```python
from build123d import *

# Parameters (mm, degrees)
BASE_FLANGE1_DEPTH = 2
HEM1_START         = -30
HEM1_DEPTH         = 10
HEM1_START_2       = 20
HEM1_2_DEPTH       = 10
SKETCH14_R         = 2
CUT_EXTRUDE1_DEPTH = 10
CHAMFER1_SIZE      = 1


# Read off the part's stored shape, not the designer's step: Hem1
# Sheet-metal steps are written as plain solids
with BuildPart() as part:
    # Sketch1 → Base-Flange1 (new body)
    with BuildSketch(Plane(origin=(0, 0, 0), x_dir=(1, 0, 0), z_dir=(0, 1, 0))):
        with BuildLine():
            Line((20, -15), (30, -15))
            Line((30, -15), (30, 12))
            ThreePointArc((30, 12), (29.121320344, 14.121320344), (27, 15))
            Line((27, 15), (-27, 15))
            ThreePointArc((-27, 15), (-29.121320344, 14.121320344), (-30, 12))
            Line((-30, 12), (-30, -15))
            Line((-30, -15), (-20, -15))
            Line((-20, -15), (-20, 2))
            ThreePointArc((-20, 2), (-19.121320344, 4.121320344), (-17, 5))
            Line((-17, 5), (17, 5))
            ThreePointArc((17, 5), (19.121320344, 4.121320344), (20, 2))
            Line((20, 2), (20, -15))
        make_face()
    extrude(amount=-BASE_FLANGE1_DEPTH)

    # Hem1 outline → Hem1 (add)
    with BuildSketch(Plane.YZ.offset(HEM1_START)):
        with BuildLine():
            Line((2.038247626, 12.343703978), (1.520609536, 10.411852325))
            ThreePointArc((1.520609536, 10.411852325), (6.518428366, 17.891616788), (-2, 15))
            Line((-2, 15), (0, 15))
            ThreePointArc((0, 15), (4.931721686, 16.67409393), (2.038247626, 12.343703978))
        make_face()
    extrude(amount=HEM1_DEPTH)

    # Hem1 2 outline → Hem1 2 (add)
    with BuildSketch(Plane.YZ.offset(HEM1_START_2)):
        with BuildLine():
            Line((2.038247626, 12.343703978), (1.520609536, 10.411852325))
            ThreePointArc((1.520609536, 10.411852325), (6.518428366, 17.891616788), (-2, 15))
            Line((-2, 15), (0, 15))
            ThreePointArc((0, 15), (4.931721686, 16.67409393), (2.038247626, 12.343703978))
        make_face()
    extrude(amount=HEM1_2_DEPTH)

    # Sketch14 → Cut-Extrude1 (cut)
    with BuildSketch(Plane(origin=(0, 0, 0), x_dir=(1, 0, 0), z_dir=(0, 1, 0))):
        with Locations(Location((0, 10, 0), (0, 0, 270))):
            Circle(SKETCH14_R)
        with Locations(Location((-25, -5, 0), (0, 0, 270))):
            Circle(SKETCH14_R)
        with Locations(Location((25, -5, 0), (0, 0, 270))):
            Circle(SKETCH14_R)
    extrude(amount=-CUT_EXTRUDE1_DEPTH, mode=Mode.SUBTRACT)

    # Chamfer1
    chamfer1_edges = [part.edges().sort_by_distance(p)[0] for p in [
        (0, 0, -12),
        (-25, 0, 3),
        (25, 0, 3),
    ]]
    chamfer(chamfer1_edges, length=CHAMFER1_SIZE)


solid = part.part
```
The model under review builds one solid part; all positions refer to its coordinate system, in mm. A direction names the side the tool comes from. Round coordinates to 2 decimals unless told otherwise and drop trailing zeros. Write each loop counter-clockwise with the first axis right and the second up, starting at its lowest first coordinate (ties: lowest second). Pieces come first, ordered by that corner, then holes. Notation, with made-up numbers: (47.5, 13) - (87.5, 13) arc R10 cw to (87.5, 18) - close; hole circle Ø2 at (33.5, -6.75). An arc over 180 degrees is marked (long way). Use one line per item in the form item = value.
Q1. Draft analysis for pull direction X (two halves, no side actions). For faces 3 (the flat face through (-25.07, 1.783, 11.391)), 4 (the flat face through (-30, -0.4, 8.7)), 5 (the flat face through (-20, 2, 11)), state which applies: +X half, -X half, draft (parallel to the pull), parting line (faces both ways), or undercut.
Answer key:
face_3 = draft
face_4 = -X half
face_5 = undercut
Q2. Consider section A-A (z = 5). State the section outline as (x, y) points, and give its area (3 significant figures).
Answer key:
outline = (-30, -2) - (-27, -2) - (-27, -1) - (-28, 0) - (-30, 0) - close; (-23, -2) - (-20, -2) - (-20, 0) - (-22, 0) - (-23, -1) - close; (20, -2) - (23, -2) - (23, -1) - (22, 0) - (20, 0) - close; (27, -2) - (30, -2) - (30, 0) - (28, 0) - (27, -1) - close
area = 22.0 mm2
Q3. Insertion check: pin 1 Ø1.5 at (x, z) = (7.5, -2.5) entering from -Y; pin 2 Ø5 at (x, z) = (6.5, -3.5) entering from +Y; pin 3 Ø1.6 at (x, y) = (-0.5, -1.5) entering from +Z; pin 4 Ø4.5 at (x, z) = (0, -10) entering from +Y. Each pin has a flat end and moves straight along its axis. Give the tip position at first contact, or say it passes through.
Answer key:
pin_1 = through
pin_2 = 0
pin_3 = -5
pin_4 = -0.75
Q4. Consider section C-C (y = 2.75). State the section outline as (x, z) points, and give its area (3 significant figures).
Answer key:
outline = (-30, 10.25) - (-20, 10.25) - (-20, 12.25) - (-30, 12.25) - close; (-30, 17.75) - (-20, 17.75) - (-20, 19.75) - (-30, 19.75) - close; (20, 10.25) - (30, 10.25) - (30, 12.25) - (20, 12.25) - close; (20, 17.75) - (30, 17.75) - (30, 19.75) - (20, 19.75) - close
area = 80.0 mm2
Q5. Consider section B-B (x = 25). State the section outline as (y, z) points.
Answer key:
outline = (-2, -15) - (0, -15) - (0, 2) - (-1, 3) - (-2, 3) - close; (-2, 7) - (-1, 7) - (0, 8) - (0, 15) arc R2.75 cw (long way) to (2.04, 12.34) - (1.52, 10.41) arc R4.75 ccw (long way) to (-2, 15) - close
Q6. For line 1 (X direction, y = -1.3, z = 5); line 2 (X direction, y = -1.45, z = -10); line 3 (X direction, y = 7, z = 13), list the stretches that pass through material, from the lowest coordinate up. Write a range as [from, to].
Answer key:
line_1 = [-30, -27], [-23, -20], [20, 23], [27, 30]
line_2 = [-30, -2], [2, 30]
line_3 = [-30, -20], [20, 30]
Q7. Tool access review of faces 1 (the flat face through (0, -1, -15)), 2 (the flat face through (20, 2, 11)): name each direction out of +Z, -Z, +X, -X, +Y, -Y from which nothing blocks a thin tool from reaching the whole face with its end or side.
Answer key:
face_1 = -Z, +X, -X, +Y, -Y
face_2 = +Z, +Y, -Y
Q8. Consider section D-D (z = -10). State the section outline as (x, y) points, and give its area (3 significant figures).
Answer key:
outline = (-30, -2) - (-2, -2) - (-2, -1) - (-3, 0) - (-30, 0) - close; (2, -2) - (30, -2) - (30, 0) - (3, 0) - (2, -1) - close
area = 111 mm2
